Read the model definition and answer for the solid it produces. Units are mm, in the model's axes. A direction names the side the tool comes from. Coordinates: 2 decimals unless noted, no trailing zeros. Order: outer loops, then holes, each group sorted by start corner. A loop starts at its lowest first (then second) coordinate and runs counter-clockwise, first axis right, second up. Notation, with made-up numbers: (-17, 38) -> (22, 38) arc R26 ccw to (22, 68) -> close; hole circle Ø4 at (9.25, 24.25). An arc over 180 degrees is marked (long way). Use CSV: the item, a comma, the result in double quotes.
```python
from build123d import *

# Parameters (mm, degrees)
SKIZZE2_W                            = 100
SKIZZE2_H                            = 39.364160046
AUFSATZ_LINEAR_AUSTRAGEN1_DEPTH      = 30
SCHNITT_LINEAR_AUSTRAGEN1_DEPTH      = 40
SCHNITT_LINEAR_AUSTRAGEN1_DEPTH_BACK = 40
SKIZZE10_R                           = 5
SKIZZE17_R                           = 1.4
SCHNITT_LINEAR_AUSTRAGEN2_DEPTH      = 103.710939516
SKIZZE24_R                           = 1.55
SCHNITT_LINEAR_AUSTRAGEN4_DEPTH      = 112.577493681
SKIZZE37_R                           = 0.736865544
SCHNITT_LINEAR_AUSTRAGEN9_DEPTH      = 112.577493681
SKIZZE40_R                           = 2.1
SCHNITT_LINEAR_AUSTRAGEN10_DEPTH     = 6
SKIZZE42_R                           = 0.75
SCHNITT_LINEAR_AUSTRAGEN12_DEPTH     = 10
VERRUNDUNG1_R                        = 1
SKIZZE46_R                           = 2.85
SCHNITT_LINEAR_AUSTRAGEN15_DEPTH     = 10
SCHNITT_LINEAR_START                 = -5
SCHNITT_LINEAR_AUSTRAGEN25_DEPTH     = 2.7
LINEARES_MUSTER1_COUNT               = 5
LINEARES_MUSTER1_PITCH               = 17
SPIEGELN2_COPY_1_SKETCH_R            = 2.85
SPIEGELN2_COPY_1_DEPTH               = 10
SPIEGELN2_COPY_2_SKETCH_R            = 2.85
SPIEGELN2_COPY_2_DEPTH               = 10
SPIEGELN2_COPY_3_SKETCH_R            = 2.85
SPIEGELN2_COPY_3_DEPTH               = 10
SPIEGELN2_COPY_4_SKETCH_R            = 2.85
SPIEGELN2_COPY_4_DEPTH               = 10
SPIEGELN2_START                      = -5
SPIEGELN2_COPY_5_DEPTH               = 2.7
SPIEGELN2_COPY_6_DEPTH               = 2.7
SPIEGELN2_COPY_7_DEPTH               = 2.7
SPIEGELN2_COPY_8_DEPTH               = 2.7
SCHNITT_LINEAR_START_2               = -10
SKIZZE51_R                           = 1.55
SCHNITT_LINEAR_AUSTRAGEN26_DEPTH     = 10
SKIZZE52_W                           = 15
SKIZZE52_H                           = 39.364160046
SCHNITT_LINEAR_AUSTRAGEN27_DEPTH     = 112.577493681


with BuildPart() as part:
    # Skizze2 → Aufsatz-Linear austragen1 (new body)
    with BuildSketch(Plane.XY):
        with Locations((50, 19.682080023)):
            Rectangle(SKIZZE2_W, SKIZZE2_H)
    extrude(amount=AUFSATZ_LINEAR_AUSTRAGEN1_DEPTH)

    # Skizze10 → Schnitt-Linear austragen1 (cut, two sides: drawn at the far end of the back side and taken through both)
    with BuildSketch(Plane.ZY.offset(-50).offset(-SCHNITT_LINEAR_AUSTRAGEN1_DEPTH_BACK)):
        with Locations((14.945770016, 20.027045739)):
            Circle(SKIZZE10_R)
    extrude(amount=SCHNITT_LINEAR_AUSTRAGEN1_DEPTH + SCHNITT_LINEAR_AUSTRAGEN1_DEPTH_BACK, mode=Mode.SUBTRACT)

    # Skizze17 → Schnitt-Linear austragen2 (cut, through all)
    with BuildSketch(Plane.ZY.offset(-90)):
        with Locations((14.945770016, 20.027045739)):
            Circle(SKIZZE17_R)
    schnitt_linear_austragen2 = extrude(amount=-SCHNITT_LINEAR_AUSTRAGEN2_DEPTH, mode=Mode.SUBTRACT)

    # Spiegeln1: Schnitt-Linear austragen2 across plane
    add(schnitt_linear_austragen2.mirror(Plane.ZY.offset(-50)), mode=Mode.SUBTRACT)

    # Skizze24 → Schnitt-Linear austragen4 (cut, through all)
    with BuildSketch(Plane.XY.offset(30)):
        with Locations((16, 31.364160046)):
            Circle(SKIZZE24_R)
        with Locations((33, 31.364160046)):
            Circle(SKIZZE24_R)
        with Locations((50, 31.364160046)):
            Circle(SKIZZE24_R)
        with Locations((67, 31.364160046)):
            Circle(SKIZZE24_R)
        with Locations((84, 31.364160046)):
            Circle(SKIZZE24_R)
    schnitt_linear_austragen4 = extrude(amount=-SCHNITT_LINEAR_AUSTRAGEN4_DEPTH, mode=Mode.SUBTRACT)

    # Skizze37 → Schnitt-Linear austragen9 (cut, through all)
    with BuildSketch(Plane(origin=(100, 0, 0), x_dir=(0, 0, -1), z_dir=(1, 0, 0))):
        with Locations((-18.924590299, 18.633559666)):
            Circle(SKIZZE37_R)
    extrude(amount=-SCHNITT_LINEAR_AUSTRAGEN9_DEPTH, mode=Mode.SUBTRACT)

    # Skizze40 → Schnitt-Linear austragen10 (cut)
    with BuildSketch(Plane(origin=(100, 0, 0), x_dir=(0, 0, -1), z_dir=(1, 0, 0))):
        with Locations((-18.924590299, 18.633559666)):
            Circle(SKIZZE40_R)
    extrude(amount=-SCHNITT_LINEAR_AUSTRAGEN10_DEPTH, mode=Mode.SUBTRACT)

    # Skizze42 → Schnitt-Linear austragen12 (cut)
    with BuildSketch(Plane.ZY):
        with Locations((10.86415918, 18.842582577)):
            Circle(SKIZZE42_R)
    extrude(amount=-SCHNITT_LINEAR_AUSTRAGEN12_DEPTH, mode=Mode.SUBTRACT)

    # Verrundung1
    verrundung1_edges = [part.edges().sort_by_distance(p)[0] for p in [
        (94, 18.633559666, 19.661455843),
    ]]
    fillet(verrundung1_edges, radius=VERRUNDUNG1_R)

    # Skizze46 → Schnitt-Linear austragen15 (cut)
    with BuildSketch(Plane(origin=(0, 0, 0), x_dir=(-1, 0, 0), z_dir=(0, 0, -1))):
        with Locations((-84, 31.364160046)):
            Circle(SKIZZE46_R)
    schnitt_linear_austragen15 = extrude(amount=-SCHNITT_LINEAR_AUSTRAGEN15_DEPTH, mode=Mode.SUBTRACT)

    # Skizze50 → Schnitt-Linear austragen25 (cut)
    with BuildSketch(Plane.XY.offset(30).offset(SCHNITT_LINEAR_START)):
        Polygon((81.15, 33.009608314), (81.15, 39.364160046), (86.85, 39.364160046), (86.85, 33.009608314), (86.85, 29.718711779), (84, 28.073263512), (81.15, 29.718711779), align=None)
    schnitt_linear_austragen25 = extrude(amount=-SCHNITT_LINEAR_AUSTRAGEN25_DEPTH, mode=Mode.SUBTRACT)

    # Lineares Muster1: Schnitt-Linear austragen15, Schnitt-Linear austragen25 ×5
    with Locations(*[(-i * LINEARES_MUSTER1_PITCH, 0, 0) for i in range(1, LINEARES_MUSTER1_COUNT)]):
        add(schnitt_linear_austragen15, mode=Mode.SUBTRACT)
        add(schnitt_linear_austragen25, mode=Mode.SUBTRACT)

    # Spiegeln2: Schnitt-Linear austragen15, Schnitt-Linear austragen25 across plane
    add(schnitt_linear_austragen15.mirror(Plane.ZX.offset(19.764160046)), mode=Mode.SUBTRACT)
    add(schnitt_linear_austragen25.mirror(Plane.ZX.offset(19.764160046)), mode=Mode.SUBTRACT)

    # Spiegeln2 copy 1 sketch → Spiegeln2 copy 1 (cut)
    with BuildSketch(Plane(origin=(-17, 39.528320093, 0), x_dir=(-1, 0, 0), z_dir=(0, 0, -1))):
        with Locations((-84, -31.364160046)):
            Circle(SPIEGELN2_COPY_1_SKETCH_R)
    extrude(amount=-SPIEGELN2_COPY_1_DEPTH, mode=Mode.SUBTRACT)

    # Spiegeln2 copy 2 sketch → Spiegeln2 copy 2 (cut)
    with BuildSketch(Plane(origin=(-34, 39.528320093, 0), x_dir=(-1, 0, 0), z_dir=(0, 0, -1))):
        with Locations((-84, -31.364160046)):
            Circle(SPIEGELN2_COPY_2_SKETCH_R)
    extrude(amount=-SPIEGELN2_COPY_2_DEPTH, mode=Mode.SUBTRACT)

    # Spiegeln2 copy 3 sketch → Spiegeln2 copy 3 (cut)
    with BuildSketch(Plane(origin=(-51, 39.528320093, 0), x_dir=(-1, 0, 0), z_dir=(0, 0, -1))):
        with Locations((-84, -31.364160046)):
            Circle(SPIEGELN2_COPY_3_SKETCH_R)
    extrude(amount=-SPIEGELN2_COPY_3_DEPTH, mode=Mode.SUBTRACT)

    # Spiegeln2 copy 4 sketch → Spiegeln2 copy 4 (cut)
    with BuildSketch(Plane(origin=(-68, 39.528320093, 0), x_dir=(-1, 0, 0), z_dir=(0, 0, -1))):
        with Locations((-84, -31.364160046)):
            Circle(SPIEGELN2_COPY_4_SKETCH_R)
    extrude(amount=-SPIEGELN2_COPY_4_DEPTH, mode=Mode.SUBTRACT)

    # Spiegeln2 copy 5 sketch → Spiegeln2 copy 5 (cut)
    with BuildSketch(Plane(origin=(-17, 39.528320093, 30), x_dir=(1, 0, 0), z_dir=(0, 0, 1)).offset(SPIEGELN2_START)):
        Polygon((81.15, -33.009608314), (81.15, -39.364160046), (86.85, -39.364160046), (86.85, -33.009608314), (86.85, -29.718711779), (84, -28.073263512), (81.15, -29.718711779), align=None)
    extrude(amount=-SPIEGELN2_COPY_5_DEPTH, mode=Mode.SUBTRACT)

    # Spiegeln2 copy 6 sketch → Spiegeln2 copy 6 (cut)
    with BuildSketch(Plane(origin=(-34, 39.528320093, 30), x_dir=(1, 0, 0), z_dir=(0, 0, 1)).offset(SPIEGELN2_START)):
        Polygon((81.15, -33.009608314), (81.15, -39.364160046), (86.85, -39.364160046), (86.85, -33.009608314), (86.85, -29.718711779), (84, -28.073263512), (81.15, -29.718711779), align=None)
    extrude(amount=-SPIEGELN2_COPY_6_DEPTH, mode=Mode.SUBTRACT)

    # Spiegeln2 copy 7 sketch → Spiegeln2 copy 7 (cut)
    with BuildSketch(Plane(origin=(-51, 39.528320093, 30), x_dir=(1, 0, 0), z_dir=(0, 0, 1)).offset(SPIEGELN2_START)):
        Polygon((81.15, -33.009608314), (81.15, -39.364160046), (86.85, -39.364160046), (86.85, -33.009608314), (86.85, -29.718711779), (84, -28.073263512), (81.15, -29.718711779), align=None)
    extrude(amount=-SPIEGELN2_COPY_7_DEPTH, mode=Mode.SUBTRACT)

    # Spiegeln2 copy 8 sketch → Spiegeln2 copy 8 (cut)
    with BuildSketch(Plane(origin=(-68, 39.528320093, 30), x_dir=(1, 0, 0), z_dir=(0, 0, 1)).offset(SPIEGELN2_START)):
        Polygon((81.15, -33.009608314), (81.15, -39.364160046), (86.85, -39.364160046), (86.85, -33.009608314), (86.85, -29.718711779), (84, -28.073263512), (81.15, -29.718711779), align=None)
    extrude(amount=-SPIEGELN2_COPY_8_DEPTH, mode=Mode.SUBTRACT)

    # Spiegeln3: Schnitt-Linear austragen4 across plane
    add(schnitt_linear_austragen4.mirror(Plane.ZX.offset(19.764160046)), mode=Mode.SUBTRACT)

    # Skizze51 → Schnitt-Linear austragen26 (cut)
    with BuildSketch(Plane.XY.offset(30).offset(SCHNITT_LINEAR_START_2)):
        with Locations((5, 34.364160046)):
            Circle(SKIZZE51_R)
        with Locations((95, 5)):
            Circle(SKIZZE51_R)
    extrude(amount=-SCHNITT_LINEAR_AUSTRAGEN26_DEPTH, mode=Mode.SUBTRACT)

    # Skizze52 → Schnitt-Linear austragen27 (cut, through all)
    with BuildSketch(Plane.ZY):
        with Locations((22.5, 19.682080023)):
            Rectangle(SKIZZE52_W, SKIZZE52_H)
    extrude(amount=-SCHNITT_LINEAR_AUSTRAGEN27_DEPTH, mode=Mode.SUBTRACT)


solid = part.part
```
Item 1: Find section D-D, the plane x = 95. Give the vertices of the cut face in (y, z), then the cut area to 3 significant figures.
Return value:
outline,"(0, 0) -> (39.36, 0) -> (39.36, 15) -> (21.43, 15) arc R1.4 cw (long way) to (18.63, 15) -> (6.55, 15) -> (6.55, 10) -> (3.45, 10) -> (3.45, 15) -> (0, 15) -> close"
area,"572 mm^2"
Item 2: A tool of negligible diameter and unlimited length cuts with its end or side. For faces 1 (the flat face through (10, 20, 13)), 2 (the flat face through (82.8, 30.1, 10)), 3 (the cylindrical face through (51.48, 31.83, 12.54)), from which of +Z, -Z, +X, -X, +Y, -Y can it reach the whole face along a straight path? Write none if from no direction.
Return value:
face 1,"+Z"
face 2,"-Z"
face 3,"+Z, -Z"
Item 3: Straight lines are drawn through the part: line 1 along Y through (x, z) = (84, 14.5); line 2 along Y through (x, z) = (67, 4.75); line 3 along X through (y, z) = (22, 12.75). For each, find the intervals that lie inside material, in ascending order.
Return value:
line 1,"y = 0 to 6.61, 9.71 to 15.05, 25.01 to 29.81, 32.91 to 39.36"
line 2,"y = 0 to 5.31, 11.01 to 28.51, 34.21 to 39.36"
line 3,"x = 0 to 10, 90 to 100"
Item 4: Find section C-C, the plane z = 6.25. Give the number of separate pieces and of enclosed holes in the cut face, then the cut area to 3 significant figures.
Return value:
separate pieces,"1"
enclosed holes,"10"
area,"3,680 mm^2"
Item 5: Each of these flat-tipped pins is pushed along its axis until it touches: P1, Ø1.5, axis at x = 94.5, y = 5, coming from the +Z side; P2, Ø3.5, axis at x = 33, y = 8.16, coming from the -Z side. Where does it stop, or does it pass through?
Return value:
P1,"stops at z = 10"
P2,"stops at z = 10"
Item 6: Find section B-B, the plane y = 23. Give the vertices of the cut face in (x, z), then the cut area to 3 significant figures.
Return value:
outline,"(0, 0) -> (100, 0) -> (100, 15) -> (90, 15) -> (90, 10.93) -> (10, 10.93) -> (10, 15) -> (0, 15) -> close"
area,"1,170 mm^2"
Item 7: The mould has two halves that part along X. Classify faces 4 (the flat face through (100, 19, 7)), 5 (the cylindrical face through (5.07, 20.059, 13.546)), 6 (the cylindrical face through (16.618, 28.582, 4.93)): +X half, -X half, draft (parallel to the pull), parting line (faces both ways), or undercut.
Return value:
face 4,"+X half"
face 5,"draft"
face 6,"undercut"
Item 8: Find section A-A, the plane x = 5. Give the vertices of the cut face in (y, z), then the cut area to 3 significant figures.
Return value:
outline,"(0, 0) -> (39.36, 0) -> (39.36, 15) -> (35.91, 15) -> (35.91, 10) -> (32.81, 10) -> (32.81, 15) -> (21.43, 15) arc R1.4 cw (long way) to (18.63, 15) -> (0, 15) -> close; hole circle Ø1.5 at (18.84, 10.86)"
area,"570 mm^2"
